Could you check a few things on this model? Use its own coordinates, in mm. A direction names the side the tool comes from. Round coordinates to 2 decimals unless told otherwise and drop trailing zeros. Write each loop counter-clockwise with the first axis right and the second up, starting at its lowest first coordinate (ties: lowest second). Pieces come first, ordered by that corner, then holes. Notation, with made-up numbers: (60, 31.5) - (118, 31.5) arc R11 cw to (118, 38.5) - close; hole circle Ø6 at (30, 46). An arc over 180 degrees is marked (long way). Write each question's results on one line, items separated by ' | '. Start each with the question number.
(1) Imagine slicing it at D-D on z = 9. Write out the boundary of the cut face in (x, y), then the cut area to 3 significant figures.
(2) On a 3-axis mill with a long thin cutter (end or side, diameter ignored), from which of +Z, -Z, +X, -X, +Y, -Y can I reach the whole of each face in a straight line? I mean faces 4 (the cylindrical face through (-0.26, -1.683, 6.549)), 5 (the flat face through (0, -4, 0)). Say none if no direction works.
(3) For P1, Ø5, axis at x = -7, z = 4, coming from the -Y side; P2, Ø5, axis at y = -11, z = 2, coming from the -X side; P3, Ø1, axis at x = 4, z = 9, coming from the +Y side, each with a flat end and sliding along its axis, tell me the tip position at first contact or that it passes through.
(4) Thinking about a two-plate mould opening in X: for faces 1 (the flat face through (-2, -5, 10)), 2 (the flat face through (0, -4, 3)), 3 (the cylindrical face through (4.61, -12.54, 3.45)), which applies, +X half, -X half, draft (parallel to the pull), parting line (faces both ways), or undercut?
(5) Imagine slicing it at A-A on x = 0. Write out the boundary of the cut face in (y, z), then the cut area to 3 significant figures.
(6) Imagine slicing it at C-C on z = 1.75. Write out the boundary of the cut face in (x, y), then the cut area to 3 significant figures.
(7) Please list where these lines run through material, in increasing order: line 1 (Y direction, x = 0, z = 7); line 2 (X direction, y = -4, z = 8.25); line 3 (Y direction, x = -0.25, z = 8.75). Write a range as [from, to].
(8) Imagine slicing it at B-B on z = 5. Write out the boundary of the cut face in (x, y), then the cut area to 3 significant figures.
```python
from build123d import *

# Parameters (mm, degrees)
SKETCH1_R           = 10
BOSS_EXTRUDE1_DEPTH = 10
FILLET1_R           = 3
SKETCH2_R           = 2
CUT_EXTRUDE1_DEPTH  = 7


with BuildPart() as part:
    # Sketch1 → Boss-Extrude1 (new body)
    with BuildSketch(Plane.XY):
        with Locations((0, -3.665819089)):
            Circle(SKETCH1_R)
    extrude(amount=BOSS_EXTRUDE1_DEPTH)

    # Fillet1
    fillet1_edges = [part.edges().sort_by_distance(p)[0] for p in [
        (-10, -3.665819089, 10),
    ]]
    fillet(fillet1_edges, radius=FILLET1_R)

    # Sketch2 → Cut-Extrude1 (cut)
    with BuildSketch(Plane.XY.offset(10)):
        with Locations((0, -3.665819089)):
            Circle(SKETCH2_R)
    extrude(amount=-CUT_EXTRUDE1_DEPTH, mode=Mode.SUBTRACT)


solid = part.part
```
Response:
1) outline: circle Ø18.47 at (0, -3.67); hole circle Ø4 at (0, -3.67) | area: 255 mm²
2) face 4: +Z | face 5: -Z, +X, -X, +Y, -Y
3) P1: y = -12.6 | P2: x = -8.75 | P3: y = 5.13
4) face 1: draft | face 2: undercut | face 3: parting line
5) outline: (-13.67, 0) - (6.33, 0) - (6.33, 7) arc R3 ccw to (3.33, 10) - (-1.67, 10) - (-1.67, 3) - (-5.67, 3) - (-5.67, 10) - (-10.67, 10) arc R3 ccw to (-13.67, 7) - close | area: 168 mm²
6) outline: circle Ø20 at (0, -3.67) | area: 314 mm²
7) line 1: [-13.67, -5.67], [-1.67, 6.33] | line 2: [-9.72, -1.97], [1.97, 9.72] | line 3: [-13.1, -5.65], [-1.68, 5.77]
8) outline: circle Ø20 at (0, -3.67); hole circle Ø4 at (0, -3.67) | area: 302 mm²
